```python
from build123d import *

# Parameters (mm, degrees)
SKETCH1_W           = 88.9
SKETCH1_H           = 95.25
SKETCH1_R           = 3.2639
BOSS_EXTRUDE1_DEPTH = 2.54
SKETCH4_R           = 2.159
BOSS_EXTRUDE2_DEPTH = 2.54


with BuildPart() as part:
    # Sketch1 → Boss-Extrude1 (new body)
    with BuildSketch(Plane.XY):
        Rectangle(SKETCH1_W, SKETCH1_H)
        with Locations((-38.1, -41.275)):
            Circle(SKETCH1_R, mode=Mode.SUBTRACT)
        with Locations((38.1, -41.275)):
            Circle(SKETCH1_R, mode=Mode.SUBTRACT)
        with Locations((38.1, 41.275)):
            Circle(SKETCH1_R, mode=Mode.SUBTRACT)
        with Locations((-38.1, 41.275)):
            Circle(SKETCH1_R, mode=Mode.SUBTRACT)
    extrude(amount=BOSS_EXTRUDE1_DEPTH)

    # Sketch4 → Boss-Extrude2 (add)
    with BuildSketch(Plane(origin=(30.48, 0, 0), x_dir=(0, 0, -1), z_dir=(1, 0, 0))):
        with BuildLine():
            Line((-2.54, 47.625), (-2.54, -47.625))
            add(Edge.make_bspline(
                [(-2.54, 47.625), (-175.26, 0), (-2.54, -47.625)],
                knots=[0, 0, 0, 1, 1, 1], degree=2))
        make_face()
        with Locations((-82.55, 0)):
            Circle(SKETCH4_R, mode=Mode.SUBTRACT)
        with Locations((-8.89, 0)):
            Circle(SKETCH4_R, mode=Mode.SUBTRACT)
    boss_extrude2 = extrude(amount=-BOSS_EXTRUDE2_DEPTH)

    # Mirror1: Boss-Extrude2 across plane
    add(boss_extrude2.mirror(Plane(origin=(0, 0, 0), x_dir=(0, 0, 1), z_dir=(1, 0, 0))))


solid = part.part
```
Source: CAD feature listing. Evaluate the final solid. Frame: model axes, mm. A direction names the side the tool comes from. Coordinates: 2 decimals unless noted, no trailing zeros. Loops run counter-clockwise (first coordinate to the right, second up) from the corner with the lowest first, then second, coordinate; pieces in that order, holes last. Notation, with made-up numbers: M 61.5,-9 L 102.5,-9 A22 ccw 102.5,4 Z; hole C 11,15.5 d9. An arc over 180 degrees is marked long. Use a Markdown table: item, result. Add a question column.
Q1. Access query for faces 1 (the flat face through (-27.94, 4, 37)), 2 (the cylindrical face through (-40.506, -39.069, 1.252)), 3 (the flat face through (37, 1, 2.54)). Directions: +Z, -Z, +X, -X, +Y, -Y. A direction counts if a zero-diameter tool reaches every point of the face in a straight line with its end or side. Return the directions, or none.
Q2. Draft query along Y for faces 4 (the flat face through (-1, 47.625, 1)), 5 (the flat face through (-30.48, 4, 37)), 6 (the cylindrical face through (29.228, -0.827, 6.896)), 7 (the cylindrical face through (39.61, 38.38, 1.25)). Return one class per face: pulls with the +Y half, pulls with the -Y half, needs draft (parallel to the pull), parting line crosses it, or undercut.
Q3. Section query B-B, the plane y = 0. State how many separate pieces and enclosed holes the cut face has, and give its area (3 significant figures).
Q4. Section query C-C, the plane x = 6. Return loops of the section in (y, z) (3 decimals).
Q5. Material intervals for L1, parallel to X at y = 3.5, z = 58; L2, parallel to Y at x = 38.1, z = 0.6 (3 decimals); L3, parallel to Z at x = -11, y = -11, sorted ascending.
Q6. Section query A-A, the plane x = 38.1. Return loops of the section in (y, z) (3 decimals), and give its area (3 significant figures).
Q7. First-contact query: pin 1 (10.5 mm diameter, centred on x = -38.1, y = 41.275, fed in from +Z); pin 2 (2 mm diameter, centred on y = 18, z = 48.5, fed in from -X); pin 3 (5 mm diameter, centred on y = 22.5, z = 69, fed in from +X); pin 4 (2.5 mm diameter, centred on y = 0, z = 8.89, fed in from +X). Flat tips, straight axial feed; report the tip coordinate or a pass-through.
Result:
| question | item | result |
|---|---|---|
| 1 | face 1 | +Z, +Y, -Y |
| 1 | face 2 | +Z, -Z |
| 1 | face 3 | +Z, +X, +Y, -Y |
| 2 | face 4 | pulls with the +Y half |
| 2 | face 5 | needs draft |
| 2 | face 6 | undercut |
| 2 | face 7 | undercut |
| 3 | separate pieces | 5 |
| 3 | enclosed holes | 0 |
| 3 | area | 621 mm2 |
| 4 | outline | M -47.625,0 L 47.625,0 L 47.625,2.54 L -47.625,2.54 Z |
| 5 | L1 | x = -30.48 to -27.94, 27.94 to 30.48 |
| 5 | L2 | y = -47.625 to -44.539, -38.011 to 38.011, 44.539 to 47.625 |
| 5 | L3 | z = 0 to 2.54 |
| 6 | outline | M -47.625,0 L -44.539,0 L -44.539,2.54 L -47.625,2.54 Z; M -38.011,0 L 38.011,0 L 38.011,2.54 L -38.011,2.54 Z; M 44.539,0 L 47.625,0 L 47.625,2.54 L 44.539,2.54 Z |
| 6 | area | 209 mm2 |
| 7 | pin 1 | stops at z = 2.54 |
| 7 | pin 2 | stops at x = -30.48 |
| 7 | pin 3 | stops at x = 30.48 |
| 7 | pin 4 | passes through |
